Input: part model. Units: mm. Frame: model coordinates. A direction names the side the tool comes from. Round coordinates to 2 decimals unless told otherwise and drop trailing zeros. Loops run counter-clockwise (first coordinate to the right, second up) from the corner with the lowest first, then second, coordinate; pieces in that order, holes last. Notation, with made-up numbers: (55, -10) - (107, -10) arc R20 ccw to (107, 24) - close; hole circle Ø3 at (-20.5, 46). An arc over 180 degrees is marked (long way). Use CSV: the item, a comma, the result in double quotes. Start each with the question number.
1. Cut plane C-C (x = 4.85). Return loops of the section in (y, z), and give its area (3 significant figures).
2. Material intervals for probe 1 along X at (y, z) = (-1.3, 42.68); probe 2 along Z at (x, y) = (6.5, -9.5); probe 3 along Y at (x, z) = (1, 10), sorted ascending. Write a range as from..to.
3. Pin query (flat end, axial travel): P1, Ø1.5, axis at x = 7, y = -6.5, coming from the -Z side; P2, Ø3, axis at x = 6, y = -5.5, coming from the -Z side; P3, Ø2, axis at x = 6.5, z = 37.5, coming from the -Y side; P4, Ø3, axis at x = 4.85, z = 7.32, coming from the +Y side. Return the tip coordinate at first contact, or that it passes through.
4. Cut plane D-D (x = 1). Return loops of the section in (y, z).
5. Access query for faces 1 (the cylindrical face through (5.331, -1.521, 41.154)), 2 (the flat face through (5, -10, 13.9)), 3 (the cylindrical face through (4.921, -1.521, 0.945)), 4 (the flat face through (3.7, -3, 44.1)), 5 (the flat face through (5, -7, 16.9)). Directions: +Z, -Z, +X, -X, +Y, -Y. A direction counts if a zero-diameter tool reaches every point of the face in a straight line with its end or side. Return the directions, or none.
6. Cut plane B-B (y = -11). Return loops of the section in (x, z).
7. Cut plane A-A (z = 7.32). Return loops of the section in (x, y).
8. Pull-direction query (Z, two-part tool) for faces 6 (the cylindrical face through (4.92, -16.04, 14.8)), 7 (the cylindrical face through (5.331, -1.521, 5.794)), 8 (the flat face through (9.7, -16, 25)); classes: +Z half, -Z half, draft (parallel to the pull), parting line (faces both ways), or undercut.
```python
from build123d import *

# Parameters (mm, degrees)
BOSS_EXTRUDE1_DEPTH = 9.7
FILLET3_R           = 3
SKETCH2_R           = 1.6
CUT_EXTRUDE1_DEPTH  = 9.7
CUT_EXTRUDE2_DEPTH  = 9.7


with BuildPart() as part:
    # Sketch1 → Boss-Extrude1 (new body)
    with BuildSketch(Plane(origin=(0, 0, 0), x_dir=(0, 0, -1), z_dir=(1, 0, 0))):
        Polygon((0, 0), (-16.9, 0), (-16.9, -13.9), (-33.1, -13.9), (-33.1, 0), (-50, 0), (-50, -3), (-36.1, -3), (-36.1, -16.9), (-13.9, -16.9), (-13.9, -3), (0, -3), align=None)
    extrude(amount=BOSS_EXTRUDE1_DEPTH)

    # Fillet3
    fillet3_edges = [part.edges().sort_by_distance(p)[0] for p in [
        (4.85, -3, 13.9),
        (4.85, -16.9, 13.9),
        (4.85, -16.9, 36.1),
        (4.85, -3, 36.1),
    ]]
    fillet(fillet3_edges, radius=FILLET3_R)

    # Sketch2 → Cut-Extrude1 (cut)
    with BuildSketch(Plane.XZ.offset(3)):
        with Locations(Location((4.85, 42.68, 0), (0, 0, 270))):
            Circle(SKETCH2_R)
        with Locations(Location((4.85, 7.32, 0), (0, 0, 270))):
            Circle(SKETCH2_R)
    extrude(amount=-CUT_EXTRUDE1_DEPTH, mode=Mode.SUBTRACT)

    # Sketch3 → Cut-Extrude2 (cut)
    with BuildSketch(Plane.XZ.offset(3)):
        with BuildLine():
            Line((0, 0), (9.7, 0))
            Line((9.7, 0), (9.7, 2.2))
            ThreePointArc((9.7, 2.2), (4.85, 0.945141508), (0, 2.2))
            Line((0, 2.2), (0, 0))
        make_face()
        with BuildLine():
            Line((0, 47.8), (0, 50))
            Line((0, 50), (9.7, 50))
            Line((9.7, 50), (9.7, 47.8))
            ThreePointArc((9.7, 47.8), (4.85, 49.054858492), (0, 47.8))
        make_face()
    extrude(amount=-CUT_EXTRUDE2_DEPTH, mode=Mode.SUBTRACT)


solid = part.part
```
Established:
1,outline,"(-16.9, 16.9) arc R3 ccw to (-13.9, 13.9) - (-6, 13.9) arc R3 cw to (-3, 10.9) - (-3, 8.92) - (0, 8.92) - (0, 16.9) - (-13.9, 16.9) - (-13.9, 33.1) - (0, 33.1) - (0, 41.08) - (-3, 41.08) - (-3, 39.1) arc R3 cw to (-6, 36.1) - (-13.9, 36.1) arc R3 ccw to (-16.9, 33.1) - close; (-3, 0.95) - (0, 0.95) - (0, 5.72) - (-3, 5.72) - close; (-3, 44.28) - (0, 44.28) - (0, 49.05) - (-3, 49.05) - close"
1,area,"209 mm2"
2,probe 1,"x = 0..3.25, 6.45..9.7"
2,probe 2,"z = 13.9..16.9, 33.1..36.1"
2,probe 3,"y = -3..0"
3,P1,"stops at z = 13.89"
3,P2,"stops at z = 13.14"
3,P3,"stops at y = -4.5"
3,P4,"passes through"
4,outline,"(-16.9, 16.9) arc R3 ccw to (-13.9, 13.9) - (-6, 13.9) arc R3 cw to (-3, 10.9) - (-3, 1.72) - (0, 1.72) - (0, 16.9) - (-13.9, 16.9) - (-13.9, 33.1) - (0, 33.1) - (0, 48.28) - (-3, 48.28) - (-3, 39.1) arc R3 cw to (-6, 36.1) - (-13.9, 36.1) arc R3 ccw to (-16.9, 33.1) - close"
5,face 1,"+Y, -Y"
5,face 2,"-Z, +X, -X, -Y"
5,face 3,"-Z, +Y, -Y"
5,face 4,"+Z, +X, -X, -Y"
5,face 5,"+X, -X, +Y"
6,outline,"(0, 13.9) - (9.7, 13.9) - (9.7, 16.9) - (0, 16.9) - close; (0, 33.1) - (9.7, 33.1) - (9.7, 36.1) - (0, 36.1) - close"
7,outline,"(0, -3) - (3.25, -3) - (3.25, 0) - (0, 0) - close; (6.45, -3) - (9.7, -3) - (9.7, 0) - (6.45, 0) - close"
8,face 6,"-Z half"
8,face 7,"undercut"
8,face 8,"draft"
